Build history of the part. All positions in model axes, mm. Face numbers are marked on the shaded views. Give positions to 0.01 mm unless a question says otherwise; leave off trailing zeros. Order: outer loops, then holes, each group sorted by start corner. A loop starts at its lowest first (then second) coordinate and runs counter-clockwise, first axis right, second up. Notation, with made-up numbers: (-3.5, 89.5) - (5.5, 89.5) arc R28 ccw to (5.5, 116.5) - close; hole circle Ø8 at (-25.75, 49.25). An arc over 180 degrees is marked (long way). Write each question's results on one line, items separated by ' | '. Start each with the question number.
from build123d import *

# Parameters (mm, degrees)
CROQUIS1_R              = 3
SALIENTE_EXTRUIR1_DEPTH = 8
SALIENTE_EXTRUIR2_DEPTH = 1
CROQUIS3_R              = 4
SALIENTE_EXTRUIR3_DEPTH = 33
SALIENTE_EXTRUIR5_START = -5
CROQUIS6_R              = 5
SALIENTE_EXTRUIR5_DEPTH = 20
CROQUIS7_R              = 3.75
REDONDEO3_R             = 3.75


with BuildPart() as part:
    # Croquis1 → Saliente-Extruir1 (new body)
    with BuildSketch(Plane.XY):
        Circle(CROQUIS1_R)
    extrude(amount=SALIENTE_EXTRUIR1_DEPTH)

    # Croquis2 → Saliente-Extruir2 (add)
    with BuildSketch(Plane(origin=(0, 0, 0), x_dir=(-1, 0, 0), z_dir=(0, 0, -1))):
        Polygon((4.42226819, 2.728285919), (-0.151630819, 5.193939554), (-4.573899009, 2.465653636), (-4.42226819, -2.728285919), (0.151630819, -5.193939554), (4.573899009, -2.465653636), align=None)
    extrude(amount=SALIENTE_EXTRUIR2_DEPTH)

    # Croquis3 → Saliente-Extruir3 (add)
    with BuildSketch(Plane(origin=(0, 0, -1), x_dir=(-1, 0, 0), z_dir=(0, 0, -1))):
        Circle(CROQUIS3_R)
    extrude(amount=SALIENTE_EXTRUIR3_DEPTH)

    # Croquis6 → Saliente-Extruir5 (add)
    with BuildSketch(Plane(origin=(0, 0, -34), x_dir=(-1, 0, 0), z_dir=(0, 0, -1)).offset(SALIENTE_EXTRUIR5_START)):
        Circle(CROQUIS6_R)
    extrude(amount=SALIENTE_EXTRUIR5_DEPTH)

    # Croquis7 → section 1 of recubrir2
    with BuildSketch(Plane(origin=(0, 0, -105), x_dir=(-1, 0, 0), z_dir=(0, 0, -1)), mode=Mode.PRIVATE) as recubrir2_s1:
        Circle(CROQUIS7_R)
    # loft up to a face of the part (recubrir2)
    loft([Face(Wire([part.edges().sort_by_distance((3.42273553, 3.644843137, -49))[0]])), recubrir2_s1.sketch])

    # Redondeo3
    redondeo3_edges = [part.edges().sort_by_distance(p)[0] for p in [
        (3.75, 0, -105),
    ]]
    fillet(redondeo3_edges, radius=REDONDEO3_R)


solid = part.part
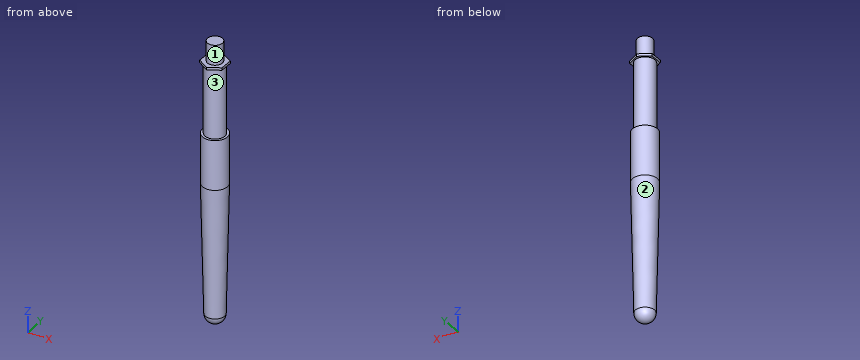
Item 1: Cut at B-B, the plane z = -58.5. List the corners of the cut face in (x, y).
Item 2: Cut at A-A, the plane z = -44. List the corners of the cut face in (x, y), then the cut area to 3 significant figures.
Item 3: Flat gauge pins, fed straight in: pin 1 Ø1.5 at (x, z) = (2, -71) entering from +Y; pin 2 Ø6 at (x, z) = (-2.5, -42) entering from +Y; pin 3 Ø3 at (x, y) = (-3, -2) entering from -Z. Where does each tip first touch, or does it go through?
Item 4: Two-plate mould, pull along Z, no slides. Class the marked faces 1, 2 and 3: +Z half, -Z half, draft (parallel to the pull), parting line (faces both ways), or undercut.
Item 5: Probe line 1 along X through (y, z) = (-2.75, -90); line 2 along X through (y, z) = (0.25, -94); line 3 along Y through (x, z) = (2, -48.5). List the from-to ranges inside material, lowest first. Write a range as from..to.
Values found:
1) outline: circle Ø9.58 at (0, 0)
2) outline: circle Ø10 at (0, 0) | area: 78.5 mm2
3) pin 1: stops at y = 4.33 | pin 2: stops at y = 5 | pin 3: stops at z = -104.41
4) face 1: draft | face 2: -Z half | face 3: undercut
5) line 1: x = -3.02..3.02 | line 2: x = -3.99..3.99 | line 3: y = -4.58..4.58
